```python
from build123d import *

# Parameters (mm, degrees)
CROQUIS1_W                   = 70
CROQUIS1_H                   = 17.5
SALIENTE_EXTRUIR1_DEPTH      = 4.2
CROQUIS2_W                   = 8.5
CROQUIS2_H                   = 13.5
CORTAR_EXTRUIR1_DEPTH        = 3
CORTAR_EXTRUIR2_DEPTH        = 2.2
SALIENTE_EXTRUIR2_DEPTH      = 3.2
CROQUIS5_R                   = 6.5
CORTAR_EXTRUIR3_DEPTH        = 4
CROQUIS6_W                   = 3.5
CROQUIS6_H                   = 6.5
CORTAR_EXTRUIR4_DEPTH        = 1
CROQUIS7_W                   = 14
CROQUIS7_H                   = 2
CORTAR_EXTRUIR5_DEPTH        = 1
CORTAR_EXTRUIR6_DEPTH        = 4
CROQUIS9_W                   = 3.489148649
CROQUIS9_H                   = 7.1
SALIENTE_EXTRUIR3_DEPTH      = 2
SALIENTE_EXTRUIR3_DEPTH_BACK = 1


with BuildPart() as part:
    # Croquis1 → Saliente-Extruir1 (new body)
    with BuildSketch(Plane(origin=(0, 0, 0), x_dir=(1, 0, 0), z_dir=(0, 1, 0))):
        with Locations((2.27027027, -4.304054054)):
            Rectangle(CROQUIS1_W, CROQUIS1_H)
    extrude(amount=SALIENTE_EXTRUIR1_DEPTH)

    # Croquis2 → Cortar-Extruir1 (cut)
    with BuildSketch(Plane(origin=(0, 4.2, 0), x_dir=(1, 0, 0), z_dir=(0, 1, 0))):
        with Locations((33.02027027, -4.304054054)):
            Rectangle(CROQUIS2_W, CROQUIS2_H)
        with Locations((-28.47972973, -4.304054054)):
            Rectangle(CROQUIS2_W, CROQUIS2_H)
    extrude(amount=-CORTAR_EXTRUIR1_DEPTH, mode=Mode.SUBTRACT)

    # Croquis3 → Cortar-Extruir2 (cut, through all)
    with BuildSketch(Plane(origin=(0, 1.2, 0), x_dir=(1, 0, 0), z_dir=(0, 1, 0))):
        with BuildLine():
            Line((37.27027027, -0.304054054), (32.27027027, -0.304054054))
            add(Edge.make_bspline(
                [(32.27027027, -0.304054054), (28.823561714, -0.304054054), (29.77027027, -5.402735351)],
                knots=[0, 0, 0, 1.84904315, 1.84904315, 1.84904315], degree=2, weights=[1, 0.602216604, 1]))
            add(Edge.make_bspline(
                [(29.77027027, -5.402735351), (30.308978827, -8.304054054), (32.27027027, -8.304054054)],
                knots=[4.990635803, 4.990635803, 4.990635803, 6.283185307, 6.283185307, 6.283185307], degree=2, weights=[1, 0.798332739, 1]))
            Line((32.27027027, -8.304054054), (37.27027027, -8.304054054))
            Line((37.27027027, -8.304054054), (37.27027027, -0.304054054))
        make_face()
        with BuildLine():
            Line((-32.72972973, -0.304054054), (-27.72972973, -0.304054054))
            add(Edge.make_bspline(
                [(-25.22972973, -4.304054054), (-25.22972973, -0.304054054), (-27.72972973, -0.304054054)],
                knots=[4.71238898, 4.71238898, 4.71238898, 6.283185307, 6.283185307, 6.283185307], degree=2, weights=[1, 0.707106781, 1]))
            add(Edge.make_bspline(
                [(-27.72972973, -8.304054054), (-25.22972973, -8.304054054), (-25.22972973, -4.304054054)],
                knots=[3.141592654, 3.141592654, 3.141592654, 4.71238898, 4.71238898, 4.71238898], degree=2, weights=[1, 0.707106781, 1]))
            Line((-27.72972973, -8.304054054), (-32.72972973, -8.304054054))
            Line((-32.72972973, -8.304054054), (-32.72972973, -0.304054054))
        make_face()
    extrude(amount=-CORTAR_EXTRUIR2_DEPTH, mode=Mode.SUBTRACT)

    # Croquis4 → Saliente-Extruir2 (add)
    with BuildSketch(Plane(origin=(0, 4.2, 0), x_dir=(1, 0, 0), z_dir=(0, 1, 0))):
        Polygon((-24.22972973, 0.945945946), (0.77027027, 0.945945946), (0.77027027, -3.054054054), (2.77027027, -3.054054054), (2.77027027, 0.945945946), (28.77027027, 0.945945946), (28.77027027, -9.554054054), (2.77027027, -9.554054054), (2.77027027, -6.354054054), (0.77027027, -6.354054054), (0.77027027, -9.554054054), (-24.22972973, -9.554054054), align=None)
    extrude(amount=SALIENTE_EXTRUIR2_DEPTH)

    # Croquis5 → Cortar-Extruir3 (cut)
    with BuildSketch(Plane.XZ):
        with Locations((-14.774068223, 3.554054054)):
            Circle(CROQUIS5_R)
        with Locations((19.216382303, 3.554054054)):
            Circle(CROQUIS5_R)
    extrude(amount=-CORTAR_EXTRUIR3_DEPTH, mode=Mode.SUBTRACT)

    # Croquis6 → Cortar-Extruir4 (cut)
    with BuildSketch(Plane.XZ.offset(-4)):
        with Locations((-17.324068223, 3.554054054)):
            Rectangle(CROQUIS6_W, CROQUIS6_H)
        with Locations((-12.224068223, 3.554054054)):
            Rectangle(CROQUIS6_W, CROQUIS6_H)
        with Locations((16.712940217, 3.293189119)):
            Rectangle(CROQUIS6_W, CROQUIS6_H)
        with Locations((21.812940217, 3.293189119)):
            Rectangle(CROQUIS6_W, CROQUIS6_H)
    extrude(amount=-CORTAR_EXTRUIR4_DEPTH, mode=Mode.SUBTRACT)

    # Croquis7 → Cortar-Extruir5 (cut)
    with BuildSketch(Plane.XZ):
        with Locations((1.291935528, -0.245945946)):
            Rectangle(CROQUIS7_W, CROQUIS7_H)
        with Locations((1.291935528, 8.854054054)):
            Rectangle(CROQUIS7_W, CROQUIS7_H)
    extrude(amount=-CORTAR_EXTRUIR5_DEPTH, mode=Mode.SUBTRACT)

    # Croquis8 → Cortar-Extruir6 (cut)
    with BuildSketch(Plane.XZ):
        with BuildLine():
            Line((-5.708064472, 7.854054054), (-5.708064472, 0.754054054))
            Line((-5.708064472, 0.754054054), (8.291935528, 0.754054054))
            Line((8.291935528, 0.754054054), (12.291935528, 0.754054054))
            add(Edge.make_bspline(
                [(11.291935528, 4.304054054), (11.291935528, 0.754054054), (12.291935528, 0.754054054)],
                knots=[1.570796327, 1.570796327, 1.570796327, 3.141592654, 3.141592654, 3.141592654], degree=2, weights=[1, 0.707106781, 1]))
            add(Edge.make_bspline(
                [(12.291935528, 7.854054054), (11.291935528, 7.854054054), (11.291935528, 4.304054054)],
                knots=[0, 0, 0, 1.570796327, 1.570796327, 1.570796327], degree=2, weights=[1, 0.707106781, 1]))
            Line((12.291935528, 7.854054054), (8.291935528, 7.854054054))
            Line((8.291935528, 7.854054054), (-5.708064472, 7.854054054))
        make_face()
    extrude(amount=-CORTAR_EXTRUIR6_DEPTH, mode=Mode.SUBTRACT)

    # Croquis9 → Saliente-Extruir3 (add, two sides)
    with BuildSketch(Plane.XZ.offset(-4)) as saliente_extruir3_sk:
        with Locations((-0.252638796, 4.304054054)):
            Rectangle(CROQUIS9_W, CROQUIS9_H)
    extrude(amount=SALIENTE_EXTRUIR3_DEPTH)
    extrude(saliente_extruir3_sk.sketch, amount=-SALIENTE_EXTRUIR3_DEPTH_BACK)


solid = part.part
```
The listing builds one solid part. Answer for the finished solid, in the listing's coordinates (mm). A direction names the side the tool comes from. Coordinates: 2 decimals unless noted, no trailing zeros. Write each loop counter-clockwise with the first axis right and the second up, starting at its lowest first coordinate (ties: lowest second). Pieces come first, ordered by that corner, then holes. Notation, with made-up numbers: (31, 66) - (77, 66) arc R18 ccw to (77, 92) - close; hole circle Ø4 at (51, 42.5). An arc over 180 degrees is marked (long way). Return JSON: item names as keys, results as strings. Group by question number.
1. Which of the six approach directions +Z, -Z, +X, -X, +Y, -Y give full straight-line access (tool end or side, diameter ignored) to faces 1 (the flat face through (16, 6, -0.946)), 2 (the flat face through (0, 2, 4)), 3 (the flat face through (29, 1.2, 4)), 4 (the flat face through (-24.23, 4, 4)), 5 (the flat face through (35, 1, 8.304))?
2. A cutting plane is placed at B-B, the plane y = 3.25. Give the number of separate pieces and of enclosed holes in the cut face, plus the area to 3 significant figures.
3. A cutting plane is placed at D-D, the plane x = -17. Determine the outline of the cut face in (y, z).
4. Determine the mould class of faces 6 (the flat face through (-32.73, 2, -3)), 7 (the flat face through (-12, 6, -0.946)), 8 (the flat face through (3, 2, 7.854)), 9 (the flat face through (2.77, 6, 1)) for opening direction X: released by +X, released by -X, zero draft, split by the parting line, or undercut.
5. A cutting plane is placed at C-C, the plane x = -7.5. Determine the outline of the cut face in (y, z).
6. Straight lines are drawn through the part: L1, parallel to X at y = 4.25, z = 2; L2, parallel to X at y = 4.5, z = 4.5; L3, parallel to Z at x = -25.5, y = 1.5. For each, find the intervals that lie inside material, in ascending order.
7. A cutting plane is placed at A-A, the plane x = 5.5. Determine the outline of the cut face in (y, z), plus the area to 3 significant figures.
8. Given pin 1 (2 mm diameter, centred on x = -11.5, z = -2, fed in from +Y); pin 2 (1.8 mm diameter, centred on x = -13, z = 4, fed in from -Y); pin 3 (1.1 mm diameter, centred on x = -4, z = 5, fed in from -Y), each flat-ended and moving along its own axis, determine where each tip first touches the part or whether it passes through.
Ans:
{
 "1": {"face 1": "-Z, +X, -X, +Y", "face 2": "-Y", "face 3": "+X, +Y", "face 4": "-X, +Y", "face 5": "+X, +Y, -Y"},
 "2": {"separate pieces": "1", "enclosed holes": "4", "area": "633 mm²"},
 "3": {"outline": "(0, -4.45) - (4.2, -4.45) - (4.2, -0.95) - (7.4, -0.95) - (7.4, 9.55) - (4.2, 9.55) - (4.2, 13.05) - (0, 13.05) - (0, 9.66) - (4, 9.66) - (4, 6.8) - (5, 6.8) - (5, 0.3) - (4, 0.3) - (4, -2.55) - (0, -2.55) - close"},
 "4": {"face 6": "released by -X", "face 7": "zero draft", "face 8": "undercut", "face 9": "undercut"},
 "5": {"outline": "(0, -4.45) - (4.2, -4.45) - (4.2, -0.95) - (7.4, -0.95) - (7.4, 9.55) - (4.2, 9.55) - (4.2, 13.05) - (0, 13.05) - close"},
 "6": {"L1": "-24.23 to -19.07, -15.57 to -13.97, -10.47 to 1.49, 2.77 to 14.96, 18.46 to 20.06, 23.56 to 28.77", "L2": "-24.23 to -19.07, -15.57 to -13.97, -10.47 to 14.96, 18.46 to 20.06, 23.56 to 28.77", "L3": "-4.45 to -2.45, 11.05 to 13.05"},
 "7": {"outline": "(0, -4.45) - (4.2, -4.45) - (4.2, -0.95) - (7.4, -0.95) - (7.4, 9.55) - (4.2, 9.55) - (4.2, 13.05) - (0, 13.05) - (0, 9.85) - (1, 9.85) - (1, 7.85) - (4, 7.85) - (4, 0.75) - (1, 0.75) - (1, -1.25) - (0, -1.25) - close", "area": "74.7 mm²"},
 "8": {"pin 1": "y = 4.2", "pin 2": "y = 5", "pin 3": "y = 4"}
}
